from build123d import *


with BuildPart() as part:
    # Sketch1 → Revolve1 (revolve)
    with BuildSketch(Plane.XY, mode=Mode.PRIVATE) as revolve1_sk:
        with BuildLine():
            Line((0, 29.4), (0, 34.4))
            ThreePointArc((0, 34.4), (24.792942544, 36.311291491), (49, 42))
            Line((49, 42), (63, 42))
            Line((63, 42), (63, 22))
            Line((63, 22), (62.2, 22))
            Line((62.2, 22), (62.2, 6))
            Line((62.2, 6), (63, 6))
            Line((63, 6), (63, 0))
            Line((63, 0), (58, 0))
            Line((58, 0), (58, 6.5))
            ThreePointArc((58, 6.5), (56.5, 8), (58, 9.5))
            Line((58, 9.5), (58, 12.5))
            ThreePointArc((58, 12.5), (56.5, 14), (58, 15.5))
            Line((58, 15.5), (58, 37))
            Line((58, 37), (49, 37))
            ThreePointArc((49, 37), (24.792942544, 31.311291491), (0, 29.4))
        make_face()
    revolve(revolve1_sk.sketch.rotate(Axis((0, 0, 0), (0, 1, 0)), 90), axis=Axis((0, 0, 0), (0, 1, 0)))


solid = part.part
Can you work these out from the model? Positions are in its coordinate system, mm. A direction names the side the tool comes from. Give positions to 0.01 mm unless a question says otherwise; leave off trailing zeros. Order: outer loops, then holes, each group sorted by start corner. A loop starts at its lowest first (then second) coordinate and runs counter-clockwise, first axis right, second up. Notation, with made-up numbers: M 81,5.5 L 90,5.5 A12 cw 90,14.5 Z; hole C -39.5,-37.75 d1. An arc over 180 degrees is marked long. One line per item, written item: value.
Item 1: If we section it at C-C on x = 0: Write out the boundary of the cut face in (y, z).
Verdict:
outline: M 0,-63 L 6,-63 L 6,-62.2 L 22,-62.2 L 22,-63 L 42,-63 L 42,-49 A161.76 cw 42,49 L 42,63 L 22,63 L 22,62.2 L 6,62.2 L 6,63 L 0,63 L 0,58 L 6.5,58 A1.5 ccw 9.5,58 L 12.5,58 A1.5 ccw 15.5,58 L 37,58 L 37,49 A161.76 ccw 37,-49 L 37,-58 L 15.5,-58 A1.5 ccw 12.5,-58 L 9.5,-58 A1.5 ccw 6.5,-58 L 0,-58 Z
Item 2: If we section it at A-A on z = 0: Write out the boundary of the cut face in (x, y).
Verdict:
outline: M -63,0 L -58,0 L -58,6.5 A1.5 ccw -58,9.5 L -58,12.5 A1.5 ccw -58,15.5 L -58,37 L -49,37 A161.76 ccw 49,37 L 58,37 L 58,15.5 A1.5 ccw 58,12.5 L 58,9.5 A1.5 ccw 58,6.5 L 58,0 L 63,0 L 63,6 L 62.2,6 L 62.2,22 L 63,22 L 63,42 L 49,42 A161.76 cw -49,42 L -63,42 L -63,22 L -62.2,22 L -62.2,6 L -63,6 Z
Item 3: For pin 1 (5 mm diameter, centred on y = 26.5, z = 29.5, fed in from -X); pin 2 (12 mm diameter, centred on x = 7, z = 36.5, fed in from -Y); pin 3 (6 mm diameter, centred on x = 44.5, y = 36.5, fed in from -Z), each with a flat end and sliding along its axis, tell me the tip position at first contact or that it passes through.
Verdict:
pin 1: x = -56.92
pin 2: y = 32.43
pin 3: z = -47.4
Item 4: Please list where these lines run through material, in increasing order: line 1 (X direction, y = 21.75, z = 0); line 2 (X direction, y = 3.25, z = 0); line 3 (Y direction, x = -46, z = 33).
Verdict:
line 1: -62.2 to -58, 58 to 62.2
line 2: -63 to -58, 58 to 63
line 3: 7.43 to 8.57, 13.43 to 14.57, 37 to 42
Item 5: If we mould it in two halves opening along Z, with no side actions, what happens to faces 1 (the face through (46.4, 6, 41.7)), 2 (the face through (51.46, 26.4, -26.76)), 3 (the face through (-48, 37, 13)), 4 (the face through (23.82, 13.89, -57.46))? For each: pulls with the +Z half, pulls with the -Z half, needs draft (parallel to the pull), parting line crosses it, or undercut.
Verdict:
face 1: needs draft
face 2: undercut
face 3: undercut
face 4: parting line crosses it
Item 6: If we section it at B-B on y = 27: Write out the boundary of the cut face in (x, z).
Verdict:
outline: C 0,0 d126; hole C 0,0 d116
Item 7: For faces 5 (the face through (51, 0, -28)), 6 (the face through (51.46, 3.3, -26.76)), 7 (the face through (41.7, 22, -46.4)), which set-ups out of +Z, -Z, +X, -X, +Y, -Y let a thin tool reach every point of the face, with its end or its side?
Verdict:
face 5: +Z, -Z, +X, -X, -Y
face 6: -Y
face 7: none
